Part model, mm, in its own coordinate system. Coordinates: 2 decimals unless noted, no trailing zeros. Write each loop counter-clockwise with the first axis right and the second up, starting at its lowest first coordinate (ties: lowest second). Pieces come first, ordered by that corner, then holes. Notation, with made-up numbers: (-5.75, -17.5) -> (46.25, -17.5) arc R16 ccw to (46.25, -1.5) -> close; hole circle Ø3 at (-5.75, -38). An arc over 180 degrees is marked (long way). Write item = value, one per line. Start each with the question number.
Q1. Band-saw the part on B-B, the plane x = 35.5. List the corners of the cut face in (y, z).
Q2. Band-saw the part on A-A, the plane z = 30. List the corners of the cut face in (x, y) (3 decimals).
Q3. Pin check, flat tips, straight feed: P1, Ø12.5, axis at x = 31.5, z = 41, coming from the +Y side; P2, Ø12, axis at x = -36, z = 4.5, coming from the +Y side; P3, Ø3, axis at x = -11.5, y = 8.5, coming from the +Z side. Stop position of each tip, or through.
Q4. Band-saw the part on C-C, the plane x = 0.5. List the corners of the cut face in (y, z).
Q5. Band-saw the part on D-D, the plane y = 8. List the corners of the cut face in (x, z), plus the area to 3 significant figures.
Q6. Probe line 1 (Y direction, x = -21.5, z = -39.5); line 2 (Z direction, x = -18, y = 6.75). List the from-to ranges inside material, lowest first.
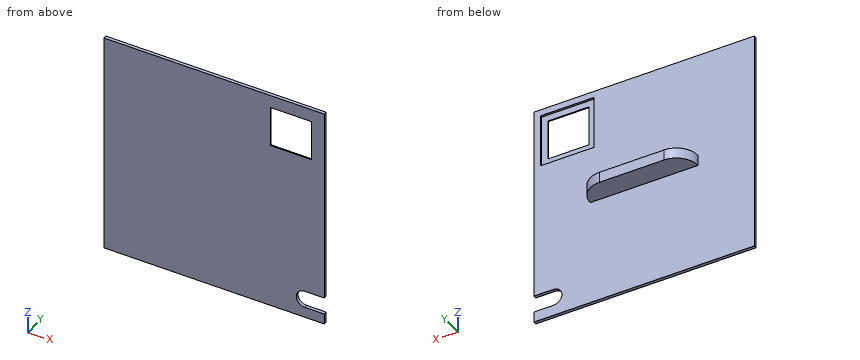
from build123d import *

# Parameters (mm, degrees)
BOSS_EXTRUDE1_DEPTH = 1.5
SKETCH2_W           = 30
SKETCH2_H           = 5
BOSS_EXTRUDE2_DEPTH = 10
SKETCH3_W           = 10
SKETCH3_H           = 5
REVOLVE_THIN1_ANGLE = 180
SKETCH5_W           = 25
SKETCH5_H           = 25
CUT_EXTRUDE1_DEPTH  = 1
SKETCH6_W           = 19
SKETCH6_H           = 19
CUT_EXTRUDE2_DEPTH  = 3


with BuildPart() as part:
    # Sketch1 → Boss-Extrude1 (new body)
    with BuildSketch(Plane(origin=(0, 0, 0), x_dir=(1, 0, 0), z_dir=(0, 1, 0))):
        with BuildLine():
            ThreePointArc((42.125, 39.560795807), (38.125, 43.560795807), (42.125, 47.560795807))
            Line((42.125, 47.560795807), (51.125, 47.560795807))
            Line((51.125, 47.560795807), (51.125, 52.560795807))
            Line((51.125, 52.560795807), (-51.125, 52.560795807))
            Line((-51.125, 52.560795807), (-51.125, -52.560795807))
            Line((-51.125, -52.560795807), (51.125, -52.560795807))
            Line((51.125, -52.560795807), (51.125, 39.560795807))
            Line((51.125, 39.560795807), (42.125, 39.560795807))
        make_face()
    extrude(amount=BOSS_EXTRUDE1_DEPTH)

    # Sketch2 → Boss-Extrude2 (add)
    with BuildSketch(Plane(origin=(0, 1.5, 0), x_dir=(1, 0, 0), z_dir=(0, 1, 0))):
        Rectangle(SKETCH2_W, SKETCH2_H)
    extrude(amount=BOSS_EXTRUDE2_DEPTH)

    # Sketch3 → Revolve-Thin1 (revolve)
    with BuildSketch(Plane(origin=(0, 1.5, 0), x_dir=(1, 0, 0), z_dir=(0, 1, 0))):
        with Locations((-20, 0)):
            Rectangle(SKETCH3_W, SKETCH3_H)
    revolve_thin1 = revolve(axis=Axis((-15, 1.5, 2.5), (0, 0, -1)), revolution_arc=REVOLVE_THIN1_ANGLE)

    # Mirror1: Revolve-Thin1 across plane
    add(revolve_thin1.mirror(Plane(origin=(0, 0, 0), x_dir=(0, 0, 1), z_dir=(1, 0, 0))))

    # Sketch5 → Cut-Extrude1 (cut)
    with BuildSketch(Plane(origin=(0, 1.5, 0), x_dir=(1, 0, 0), z_dir=(0, 1, 0))):
        with Locations((35.625, -37.060795807)):
            Rectangle(SKETCH5_W, SKETCH5_H)
    extrude(amount=-CUT_EXTRUDE1_DEPTH, mode=Mode.SUBTRACT)

    # Sketch6 → Cut-Extrude2 (cut)
    with BuildSketch(Plane(origin=(0, 0.5, 0), x_dir=(1, 0, 0), z_dir=(0, 1, 0))):
        with Locations((35.625, -37.060795807)):
            Rectangle(SKETCH6_W, SKETCH6_H)
    extrude(amount=-CUT_EXTRUDE2_DEPTH, mode=Mode.SUBTRACT)


solid = part.part
Ans:
q1.outline = (0, -52.56) -> (1.5, -52.56) -> (1.5, 24.56) -> (0.5, 24.56) -> (0.5, 27.56) -> (0, 27.56) -> close; (0, 46.56) -> (0.5, 46.56) -> (0.5, 49.56) -> (1.5, 49.56) -> (1.5, 52.56) -> (0, 52.56) -> close
q2.outline = (-51.125, 0) -> (26.125, 0) -> (26.125, 0.5) -> (23.125, 0.5) -> (23.125, 1.5) -> (-51.125, 1.5) -> close; (45.125, 0) -> (51.125, 0) -> (51.125, 1.5) -> (48.125, 1.5) -> (48.125, 0.5) -> (45.125, 0.5) -> close
q3.P1 = 0.5
q3.P2 = 1.5
q3.P3 = 2.5
q4.outline = (0, -52.56) -> (1.5, -52.56) -> (1.5, -2.5) -> (11.5, -2.5) -> (11.5, 2.5) -> (1.5, 2.5) -> (1.5, 52.56) -> (0, 52.56) -> close
q5.outline = (-22.6, -2.5) -> (22.6, -2.5) -> (22.6, 2.5) -> (-22.6, 2.5) -> close
q5.area = 226 mm2
q6.line_1 = 0 to 1.5
q6.line_2 = -2.5 to 2.5
